Design review of the part built by this model. Coordinates are the model's own, in mm. Coordinates: 2 decimals unless noted, no trailing zeros. Write each loop counter-clockwise with the first axis right and the second up, starting at its lowest first coordinate (ties: lowest second). Pieces come first, ordered by that corner, then holes. Notation, with made-up numbers: (-5.75, 32) -> (23.25, 32) arc R28 ccw to (23.25, 59) -> close; hole circle Ø3 at (6, 44.5). An arc over 180 degrees is marked (long way). Return JSON: item names as keys, results as strings. Group by question number.
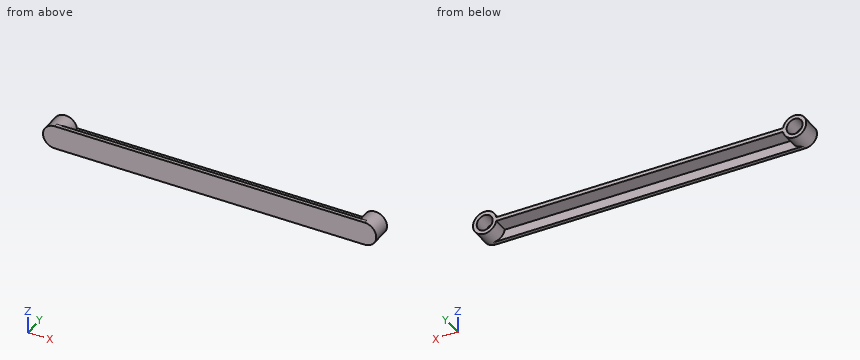
from build123d import *
from build123d.topology import SkipClean

# Parameters (mm, degrees)
BOSS_EXTRUDE1_DEPTH                  = 1.5875
SKETCH2_R                            = 4.7625
SKETCH2_R_2                          = 3.2385
BOSS_EXTRUDE2_DEPTH                  = 6.35
BOSS_EXTRUDE3_REACH                  = 158.74
BOSS_EXTRUDE3_END_RADIUS             = 4.7625
BOSS_EXTRUDE3_START                  = -25.4
SKETCH3_W                            = 1.5875
SKETCH3_H                            = 6.35
BOSS_EXTRUDE3_DIRECTION_2_REACH      = 158.74
BOSS_EXTRUDE3_DIRECTION_2_END_RADIUS = 4.7625


with BuildPart() as part:
    # Sketch1 → Boss-Extrude1 (new body)
    with BuildSketch(Plane(origin=(0, 0, 0), x_dir=(1, 0, 0), z_dir=(0, 1, 0))):
        with BuildLine():
            Line((0, -4.7625), (-126.2507, -4.7625))
            ThreePointArc((-126.2507, -4.7625), (-131.0132, 0), (-126.2507, 4.7625))
            Line((-126.2507, 4.7625), (0, 4.7625))
            ThreePointArc((0, 4.7625), (4.7625, 0), (0, -4.7625))
        make_face()
    extrude(amount=BOSS_EXTRUDE1_DEPTH)

    # Sketch2 → Boss-Extrude2 (add)
    # profile 1 of 2: a face of its own
    with SkipClean():  # the faces are left unmerged after this step: merging them gives an invalid solid
        with BuildSketch(Plane(origin=(0, 1.5875, 0), x_dir=(1, 0, 0), z_dir=(0, 1, 0))):
            with Locations(Location((-126.2507, 0, 0), (0, 0, 270))):
                Circle(SKETCH2_R)
            with Locations(Location((-126.2507, 0, 0), (0, 0, 270))):
                Circle(SKETCH2_R_2, mode=Mode.SUBTRACT)
        # profile 2 of 2: a face of its own
        with BuildSketch(Plane(origin=(0, 1.5875, 0), x_dir=(1, 0, 0), z_dir=(0, 1, 0))):
            with Locations(Location((0, 0, 0), (0, 0, 270))):
                Circle(SKETCH2_R)
            with Locations(Location((0, 0, 0), (0, 0, 270))):
                Circle(SKETCH2_R_2, mode=Mode.SUBTRACT)
        extrude(amount=BOSS_EXTRUDE2_DEPTH)

    # Boss-Extrude3: up to this cylinder (the profile starts outside it)
    with SkipClean():  # the faces are left unmerged after this step: merging them gives an invalid solid
        boss_extrude3_end = Plane(origin=(-126.2507, 4.7625, 0), z_dir=(0, -1, 0)) * Cylinder(BOSS_EXTRUDE3_END_RADIUS, 328.005, mode=Mode.PRIVATE)
        # Sketch3 → Boss-Extrude3 (add, up to the surface)
        with BuildSketch(Plane(origin=(0, 0, 0), x_dir=(0, 0, -1), z_dir=(1, 0, 0)).offset(BOSS_EXTRUDE3_START), mode=Mode.PRIVATE) as boss_extrude3_sk1:
            with Locations((0, 4.7625)):
                Rectangle(SKETCH3_W, SKETCH3_H)
        boss_extrude3_tool1 = extrude(boss_extrude3_sk1.sketch, amount=-BOSS_EXTRUDE3_REACH, mode=Mode.PRIVATE) - boss_extrude3_end
        add(boss_extrude3_tool1.solids().sort_by_distance((-25.4, 4.7625, 0))[0])
    add(part.part.scale(1), mode=Mode.REPLACE)  # the faces are merged on a copy

    # Boss-Extrude3 direction 2: up to this cylinder (the profile starts outside it)
    boss_extrude3_direction_2_end = Plane(origin=(0, 4.7625, 0), z_dir=(0, -1, 0)) * Cylinder(BOSS_EXTRUDE3_DIRECTION_2_END_RADIUS, 328.005, mode=Mode.PRIVATE)
    # Sketch3 → Boss-Extrude3 direction 2 (add, up to the surface)
    with BuildSketch(Plane(origin=(0, 0, 0), x_dir=(0, 0, -1), z_dir=(1, 0, 0)).offset(BOSS_EXTRUDE3_START), mode=Mode.PRIVATE) as boss_extrude3_direction_2_sk1:
        with Locations((0, 4.7625)):
            Rectangle(SKETCH3_W, SKETCH3_H)
    boss_extrude3_direction_2_tool1 = extrude(boss_extrude3_direction_2_sk1.sketch, amount=BOSS_EXTRUDE3_DIRECTION_2_REACH, mode=Mode.PRIVATE) - boss_extrude3_direction_2_end
    add(boss_extrude3_direction_2_tool1.solids().sort_by_distance((-25.4, 4.7625, 0))[0])


solid = part.part
Q1. We need section A-A on y = 4. Write out the cut boundary in (x, z) (1 decimal), plus the area to 3 significant figures.
Q2. For P1, Ø3, axis at x = -56, y = 6, coming from the -Z side; P2, Ø3, axis at x = -91.5, z = 0, coming from the -Y side; P3, Ø1.9, axis at x = 1, z = 0.5, coming from the +Y side; P4, Ø4, axis at y = 5.5, z = 2.5, coming from the +X side, all flat-tipped, find the tip position at first contact; note any pin that passes through.
Q3. We need section B-B on x = -61. Write out the cut boundary in (y, z), plus the area to 3 significant figures.
Q4. Wall thickness on L1, parallel to X at y = 6.5, z = 0; L2, parallel to X at y = 5, z = 0.5; L3, parallel to X at y = 6, z = -2.25: over which ranges is each line inside the solid? List them lowest first.
Findings below:
{
 "1": {"outline": "(-121.6, -0.8) -> (-4.7, -0.8) arc R4.8 ccw (long way) to (-4.7, 0.8) -> (-121.6, 0.8) arc R4.8 ccw (long way) to start; hole circle Ø6.5 at (-126.3, 0); hole circle Ø6.5 at (0, 0)", "area": "262 mm^2"},
 "2": {"P1": "stops at z = -0.79", "P2": "stops at y = 0", "P3": "stops at y = 1.59", "P4": "stops at x = 4.74"},
 "3": {"outline": "(0, -4.76) -> (1.59, -4.76) -> (1.59, -0.79) -> (7.94, -0.79) -> (7.94, 0.79) -> (1.59, 0.79) -> (1.59, 4.76) -> (0, 4.76) -> close", "area": "25.2 mm^2"},
 "4": {"L1": "x = -131.01 to -129.49, -123.01 to -3.24, 3.24 to 4.76", "L2": "x = -130.99 to -129.45, -123.05 to -3.2, 3.2 to 4.74", "L3": "x = -130.45 to -128.58, -123.92 to -122.05, -4.2 to -2.33, 2.33 to 4.2"}
}
